from build123d import *

# Parameters (mm, degrees)
SKIZZE1_W                         = 100
SKIZZE1_H                         = 20
AUFSATZ_LINEAR_AUSTRAGEN1_DEPTH   = 50
SKIZZE3_W                         = 80
SKIZZE3_H                         = 10
SCHNITT_LINEAR_AUSTRAGEN1_DEPTH   = 21
SKIZZE4_W                         = 80
SKIZZE4_H                         = 18
SCHNITT_LINEAR_AUSTRAGEN2_DEPTH   = 19
LINEAR_AUSTRAGEN_D_NN1_DEPTH      = 5
LINEAR_AUSTRAGEN_D_NN1_DEPTH_BACK = 5
SKIZZE5_W                         = 100
SKIZZE5_H                         = 20
SCHNITT_LINEAR_AUSTRAGEN3_DEPTH   = 20
VERRUNDUNG1_R                     = 3


with BuildPart() as part:
    # Skizze1 → Aufsatz-Linear austragen1 (new body)
    with BuildSketch(Plane.XY):
        with Locations((50, 10)):
            Rectangle(SKIZZE1_W, SKIZZE1_H)
    extrude(amount=AUFSATZ_LINEAR_AUSTRAGEN1_DEPTH)

    # Skizze3 → Schnitt-Linear austragen1 (cut, through all)
    with BuildSketch(Plane.XZ):
        with Locations((50, 34)):
            Rectangle(SKIZZE3_W, SKIZZE3_H)
        with Locations((50, 16)):
            Rectangle(SKIZZE3_W, SKIZZE3_H)
    extrude(amount=-SCHNITT_LINEAR_AUSTRAGEN1_DEPTH, mode=Mode.SUBTRACT)

    # Skizze4 → Schnitt-Linear austragen2 (cut)
    with BuildSketch(Plane.XZ):
        with Locations((50, 25)):
            Rectangle(SKIZZE4_W, SKIZZE4_H)
    extrude(amount=-SCHNITT_LINEAR_AUSTRAGEN2_DEPTH, mode=Mode.SUBTRACT)

    # Skizze2 → Linear-Austragen-Dünn1 (add, two sides)
    with BuildSketch(Plane.XY.offset(25)) as linear_austragen_d_nn1_sk:
        with BuildLine():
            Line((0, 20), (0, 32.789569947))
            ThreePointArc((0, 32.789569947), (4.976072473, 41.435965277), (14.95203044, 41.477342649))
            Line((14.95203044, 41.477342649), (45.04796956, 24.322657351))
            ThreePointArc((45.04796956, 24.322657351), (50, 23.010430053), (54.95203044, 24.322657351))
            Line((54.95203044, 24.322657351), (85.04796956, 41.477342649))
            ThreePointArc((85.04796956, 41.477342649), (95.023927527, 41.435965277), (100, 32.789569947))
            Line((100, 32.789569947), (100, 20))
            Line((100, 20), (99, 20))
            Line((99, 20), (99, 32.789569947))
            ThreePointArc((99, 32.789569947), (94.521534775, 40.571325744), (85.543172604, 40.608565379))
            Line((85.543172604, 40.608565379), (55.447233484, 23.453880081))
            ThreePointArc((55.447233484, 23.453880081), (50, 22.010430053), (44.552766516, 23.453880081))
            Line((44.552766516, 23.453880081), (14.456827396, 40.608565379))
            ThreePointArc((14.456827396, 40.608565379), (5.478465225, 40.571325744), (1, 32.789569947))
            Line((1, 32.789569947), (1, 20))
            Line((1, 20), (0, 20))
        make_face()
    extrude(amount=LINEAR_AUSTRAGEN_D_NN1_DEPTH)
    extrude(linear_austragen_d_nn1_sk.sketch, amount=-LINEAR_AUSTRAGEN_D_NN1_DEPTH_BACK)

    # Skizze5 → Schnitt-Linear austragen3 (cut)
    with BuildSketch(Plane(origin=(0, 0, 0), x_dir=(-1, 0, 0), z_dir=(0, 0, -1))):
        with Locations((-50, 10)):
            Rectangle(SKIZZE5_W, SKIZZE5_H)
    extrude(amount=-SCHNITT_LINEAR_AUSTRAGEN3_DEPTH, mode=Mode.SUBTRACT)

    # Verrundung1
    verrundung1_edges = [part.edges().sort_by_distance(p)[0] for p in [
        (99.5, 20, 30),
        (99, 20, 25),
        (1, 20, 25),
        (0.5, 20, 30),
    ]]
    fillet(verrundung1_edges, radius=VERRUNDUNG1_R)


solid = part.part
Build history of the part. All positions in model axes, mm. A direction names the side the tool comes from. Round coordinates to 2 decimals unless told otherwise and drop trailing zeros. Write each loop counter-clockwise with the first axis right and the second up, starting at its lowest first coordinate (ties: lowest second). Pieces come first, ordered by that corner, then holes. Notation, with made-up numbers: (-26.5, 1) -> (-15.5, 1) arc R14 ccw to (-15.5, 9) -> close; hole circle Ø10 at (-12.5, -5). An arc over 180 degrees is marked (long way). Use one line per item in the form item = value.
Q1. Drill centre lines: L1, parallel to X at y = 26.5, z = 24; L2, parallel to X at y = 9, z = 24.75; L3, parallel to Z at x = 22.5, y = 3.5. Where is each one in solid material? Low to high.
Conclusion:
L1 = 0 to 1, 39.21 to 41.23, 58.77 to 60.79, 99 to 100
L2 = 0 to 10, 90 to 100
L3 = 39 to 50
Q2. Band-saw the part on A-A, the plane z = 25.5. Write the cut outline in (x, y), then the cut area to 3 significant figures.
Conclusion:
outline = (0, 0) -> (10, 0) -> (10, 19) -> (90, 19) -> (90, 0) -> (100, 0) -> (100, 32.79) arc R10 ccw to (85.05, 41.48) -> (54.95, 24.32) arc R10 cw to (45.05, 24.32) -> (14.95, 41.48) arc R10 ccw to (0, 32.79) -> close; hole (1, 23) arc R3 ccw to (4, 20) -> (96, 20) arc R3 ccw to (99, 23) -> (99, 32.79) arc R9 ccw to (85.54, 40.61) -> (55.45, 23.45) arc R11 cw to (44.55, 23.45) -> (14.46, 40.61) arc R9 ccw to (1, 32.79) -> close
area = 629 mm²
Q3. Two-plate mould, pull along Y, no slides. Class faces 1 (the flat face through (29.79, 33.02, 25.07)), 2 (the cylindrical face through (50.08, 22.01, 25.07)), 3 (the flat face through (49, 0, 41)): released by +Y, released by -Y, zero draft, split by the parting line, or undercut.
Conclusion:
face_1 = released by +Y
face_2 = undercut
face_3 = released by -Y
Q4. Band-saw the part on B-B, the plane x = 11. Write the cut outline in (y, z).
Conclusion:
outline = (0, 39) -> (20, 39) -> (20, 50) -> (0, 50) -> close; (19, 21) -> (20, 21) -> (20, 29) -> (19, 29) -> close; (41.73, 20) -> (42.74, 20) -> (42.74, 30) -> (41.73, 30) -> close
Q5. Drop flat-ended pins along their axis: P1, Ø8, axis at x = 35.5, z = 46, coming from the +Y side; P2, Ø2, axis at x = 32, y = 6.5, coming from the -Z side; P3, Ø15, axis at x = 26, z = 30, coming from the +Y side (3 decimals). Give the stop position or say it passes through.
Conclusion:
P1 = 20
P2 = 39
P3 = 39.455
Q6. Tool access for faces 4 (the flat face through (100, 13, 32)), 5 (the flat face through (49, 19, 25)), 6 (the cylindrical face through (98.14, 20.9, 24.96)): list every direction of +Z, -Z, +X, -X, +Y, -Y with a clear straight run to the whole face (end or side of a thin tool).
Conclusion:
face_4 = +Z, -Z, +X, +Y, -Y
face_5 = -Z, -Y
face_6 = +Z, -Z
Q7. Band-saw the part on C-C, the plane z = 35.75. Write the cut outline in (x, y).
Conclusion:
outline = (0, 0) -> (10, 0) -> (10, 20) -> (0, 20) -> close; (90, 0) -> (100, 0) -> (100, 20) -> (90, 20) -> close
Q8. Band-saw the part on D-D, the plane y = 3. Write the cut outline in (x, z).
Conclusion:
outline = (0, 20) -> (10, 20) -> (10, 39) -> (90, 39) -> (90, 20) -> (100, 20) -> (100, 50) -> (0, 50) -> close
